Geometry: see drawing. Coordinates: mm, zero at the bounding-box minimum. Round coordinates to 2 decimals unless told otherwise and drop trailing zeros. Order: outer loops, then holes, each group sorted by start corner. A loop starts at its lowest first (then second) coordinate and runs counter-clockwise, first axis right, second up. Notation, with made-up numbers: (79, 88.5) -> (103, 88.5) arc R23 ccw to (103, 105.5) -> close; hole circle Ø1 at (20, 26.25). An arc over 180 degrees is marked (long way). Answer as CSV lines item,"result". Start each with the question number.
(1) Contact query for flat-ended pins moving along their axis: P1, Ø2, axis at x = 3.5, y = 3, coming from the +Z side; P2, Ø1.2, axis at x = 3, y = 2, coming from the -Z side. Output: stop coordinate, or through.
(2) Section query B-B (y = 2). Output: boundary loops of the cut face in (x, z).
(3) Line query: line 1 along Z through (x, y) = (7.5, 2.4); line 2 along Y through (x, z) = (4, 6.35); line 3 along Z through (x, y) = (17, 1.35). Output: solid intervals per line, ascending. Write a range as from..to.
(4) Section query D-D (x = 21). Output: boundary loops of the cut face in (y, z), plus the area to 3 significant figures.
(5) Section query C-C (z = 14.75). Output: boundary loops of the cut face in (x, y), plus the area to 3 significant figures.
(6) Section query A-A (x = 4). Output: boundary loops of the cut face in (y, z), plus the area to 3 significant figures.
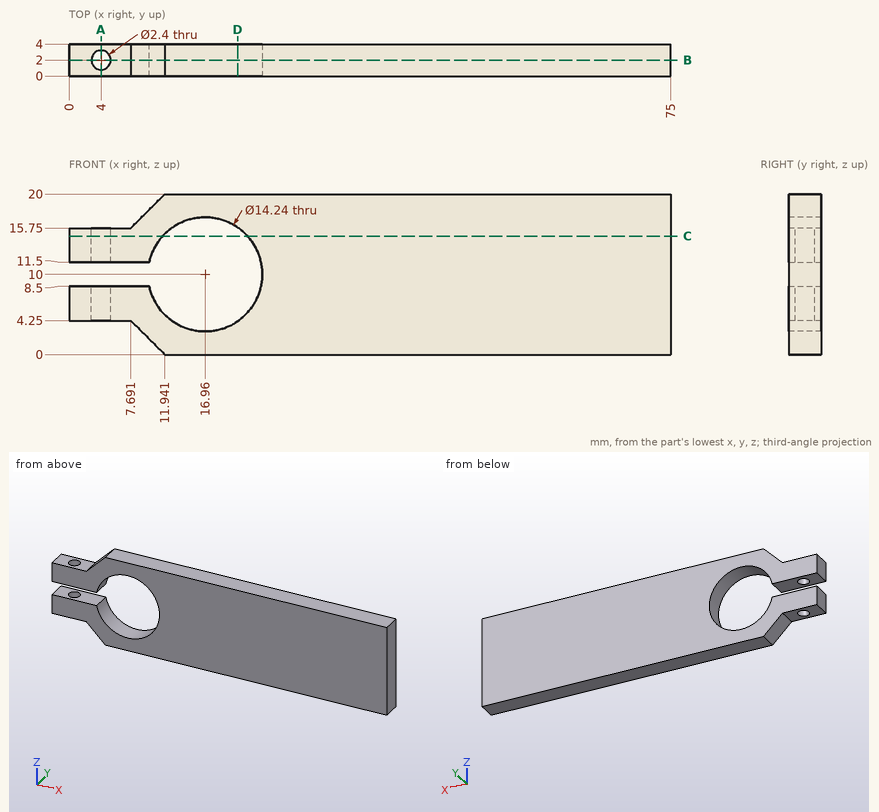
Answer block:
1,P1,"z = 15.75"
1,P2,"z = 4.25"
2,outline,"(0, 4.25) -> (2.8, 4.25) -> (2.8, 8.5) -> (0, 8.5) -> close; (0, 11.5) -> (2.8, 11.5) -> (2.8, 15.75) -> (0, 15.75) -> close; (5.2, 4.25) -> (7.69, 4.25) -> (11.94, 0) -> (75, 0) -> (75, 20) -> (11.94, 20) -> (7.69, 15.75) -> (5.2, 15.75) -> (5.2, 11.5) -> (10, 11.5) arc R7.12 cw (long way) to (10, 8.5) -> (5.2, 8.5) -> close"
3,line 1,"4.25..8.5, 11.5..15.75"
3,line 2,"0..0.8, 3.2..4"
3,line 3,"0..2.88, 17.12..20"
4,outline,"(0, 0) -> (4, 0) -> (4, 4.14) -> (0, 4.14) -> close; (0, 15.86) -> (4, 15.86) -> (4, 20) -> (0, 20) -> close"
4,area,"33.1 mm2"
5,outline,"(0, 0) -> (11.66, 0) -> (11.66, 4) -> (0, 4) -> close; (22.26, 0) -> (75, 0) -> (75, 4) -> (22.26, 4) -> close; hole circle Ø2.4 at (4, 2)"
5,area,"253 mm2"
6,outline,"(0, 4.25) -> (0.8, 4.25) -> (0.8, 8.5) -> (0, 8.5) -> close; (0, 11.5) -> (0.8, 11.5) -> (0.8, 15.75) -> (0, 15.75) -> close; (3.2, 4.25) -> (4, 4.25) -> (4, 8.5) -> (3.2, 8.5) -> close; (3.2, 11.5) -> (4, 11.5) -> (4, 15.75) -> (3.2, 15.75) -> close"
6,area,"13.6 mm2"
